CAD build for the part. Positions are in the model's coordinates, mm. A direction names the side the tool comes from. Give positions to 0.01 mm unless a question says otherwise; leave off trailing zeros. Order: outer loops, then holes, each group sorted by start corner. A loop starts at its lowest first (then second) coordinate and runs counter-clockwise, first axis right, second up.
```python
from build123d import *

# Parameters (mm, degrees)
BOSS_EXTRUDE1_DEPTH = 4.35
BOSS_EXTRUDE2_DEPTH = 22.8
CUT_EXTRUDE1_DEPTH  = 35.228241264
BOSS_EXTRUDE3_START = -12.57
SKETCH5_R           = 3.175
BOSS_EXTRUDE3_DEPTH = 12.57
SKETCH6_R           = 2.95
BOSS_EXTRUDE4_DEPTH = 2.6
CHAMFER1_SIZE       = 1.5
SKETCH7_R           = 1.5
CUT_EXTRUDE2_DEPTH  = 26.053852665
SKETCH8_R           = 1.25
CUT_EXTRUDE3_DEPTH  = 37.969425255
SKETCH9_W           = 15
SKETCH9_H           = 8.6
CUT_EXTRUDE4_DEPTH  = 25.4
CHAMFER2_SIZE       = 2.5
FILLET1_R           = 0.25


with BuildPart() as part:
    # Sketch2 → Boss-Extrude1 (new body)
    with BuildSketch(Plane(origin=(0, 0, 0), x_dir=(1, 0, 0), z_dir=(0, 1, 0))):
        with BuildLine():
            ThreePointArc((1.475, -16), (-1.7, -12.825), (-4.875, -16))
            Line((-4.875, -16), (1.475, -16))
        make_face()
        with BuildLine():
            Line((1.475, -16), (-4.875, -16))
            ThreePointArc((-4.875, -16), (-1.7, -19.175), (1.475, -16))
        make_face()
        with BuildLine():
            Line((-5.7, 15.863484846), (-5.7, 6.8))
            Line((-5.7, 6.8), (-5.7, -16))
            Line((-5.7, -16), (-4.875, -16))
            ThreePointArc((-4.875, -16), (-1.7, -12.825), (1.475, -16))
            Line((1.475, -16), (5.7, -16))
            Line((5.7, -16), (5.7, 6.8))
            Line((5.7, 6.8), (1.660846582, 14.02808686))
            ThreePointArc((1.660846582, 14.02808686), (0.248315373, 15.470627532), (-1.7, 16))
            Line((-1.7, 16), (-4.6, 16))
            ThreePointArc((-4.6, 16), (-5.154219358, 15.965740801), (-5.7, 15.863484846))
        make_face()
        with BuildLine():
            Line((-9.1, 6.8), (-5.7, 6.8))
            Line((-5.7, 6.8), (-5.7, 15.863484846))
            ThreePointArc((-5.7, 15.863484846), (-8.14964787, 14.265863337), (-9.1, 11.5))
            Line((-9.1, 11.5), (-9.1, 6.8))
        make_face()
    extrude(amount=BOSS_EXTRUDE1_DEPTH)

    # Sketch3 → Boss-Extrude2 (add)
    with BuildSketch(Plane.XY.offset(16)):
        with BuildLine():
            Line((5.7, 0.79), (-4.875, 4.092368421))
            Line((-4.875, 4.092368421), (-4.875, 2.831147875))
            ThreePointArc((-4.875, 2.831147875), (-1.758813758, 1.290370349), (-0.5, -1.95))
            ThreePointArc((-0.5, -1.95), (-0.966901247, -4.015007311), (-2.276772998, -5.678283585))
            Line((-2.276772998, -5.678283585), (5.7, 0.79))
        make_face()
        with BuildLine():
            ThreePointArc((-5.7, 2.833304297), (-7.287324911, 2.419272216), (-8.642534504, 1.494918444))
            ThreePointArc((-8.642534504, 1.494918444), (-8.890152665, -5.136032618), (-2.276772998, -5.678283585))
            ThreePointArc((-2.276772998, -5.678283585), (-0.966901247, -4.015007311), (-0.5, -1.95))
            ThreePointArc((-0.5, -1.95), (-1.758813758, 1.290370349), (-4.875, 2.831147875))
            Line((-4.875, 2.831147875), (-4.875, 0))
            Line((-4.875, 0), (-5.7, 0))
            Line((-5.7, 0), (-5.7, 2.833304297))
        make_face()
        with BuildLine():
            ThreePointArc((-4.875, 2.831147875), (-5.287453585, 2.849983603), (-5.7, 2.833304297))
            Line((-5.7, 2.833304297), (-5.7, 0))
            Line((-5.7, 0), (-4.875, 0))
            Line((-4.875, 0), (-4.875, 2.831147875))
        make_face()
        with BuildLine():
            Line((-4.875, 4.092368421), (-5.7, 4.35))
            Line((-5.7, 4.35), (-5.7, 2.833304297))
            ThreePointArc((-5.7, 2.833304297), (-5.287453585, 2.849983603), (-4.875, 2.831147875))
            Line((-4.875, 2.831147875), (-4.875, 4.092368421))
        make_face()
        with BuildLine():
            Line((-5.7, 2.833304297), (-5.7, 4.35))
            Line((-5.7, 4.35), (-8.642534504, 1.494918444))
            ThreePointArc((-8.642534504, 1.494918444), (-7.287324911, 2.419272216), (-5.7, 2.833304297))
        make_face()
    extrude(amount=-BOSS_EXTRUDE2_DEPTH)

    # Sketch4 → Cut-Extrude1 (cut, through all)
    with BuildSketch(Plane.XY.offset(16)):
        Polygon((5.7, 0), (5.7, 0.79), (4.725761535, 0), align=None)
    extrude(amount=-CUT_EXTRUDE1_DEPTH, mode=Mode.SUBTRACT)

    # Sketch5 → Boss-Extrude3 (add)
    with BuildSketch(Plane(origin=(0, 4.35, 0), x_dir=(1, 0, 0), z_dir=(0, 1, 0)).offset(BOSS_EXTRUDE3_START)):
        with Locations(Location((-1.7, -16, 0), (0, 0, 100.46651796))):
            Circle(SKETCH5_R)
    extrude(amount=BOSS_EXTRUDE3_DEPTH)

    # Sketch6 → Boss-Extrude4 (add)
    with BuildSketch(Plane.XY.offset(16)):
        with Locations((-5.3, -1.95)):
            Circle(SKETCH6_R)
    extrude(amount=BOSS_EXTRUDE4_DEPTH)

    # Chamfer1
    # the kernel refuses this chamfer: 1.5 mm, written as the material it takes off along each edge
    with BuildSketch(Plane(origin=(-5.273011582, -8.107902789, -6.8), x_dir=(0.017317974295388713, -0.021356755298707605, 0.9996219169112968), z_dir=(0.7767257469610731, 0.6298389587884852, 0))) as chamfer1_piece_1_section:
        Polygon((CHAMFER1_SIZE * 0.999621916911, -CHAMFER1_SIZE * 0.0274958766106), (-CHAMFER1_SIZE * 0.0274958766106, -CHAMFER1_SIZE * 0.999621916911), (0, 0), align=None)
    chamfer1_piece_1 = extrude(amount=16.730502051, mode=Mode.PRIVATE)
    chamfer1_piece_1 = split(chamfer1_piece_1, bisect_by=Plane(origin=(-2.677352376, 0, -6.368001428), z_dir=(0, -1, 0)), keep=Keep.TOP, mode=Mode.PRIVATE)
    add(chamfer1_piece_1, mode=Mode.SUBTRACT)

    # Sketch7 → Cut-Extrude2 (cut, through all)
    with BuildSketch(Plane(origin=(0, 4.35, 0), x_dir=(1, 0, 0), z_dir=(0, 1, 0))):
        with Locations(Location((-1.7, 12.15, 0), (0, 0, 270))):
            Circle(SKETCH7_R)
        with Locations(Location((-1.7, -16, 0), (0, 0, 270))):
            Circle(SKETCH7_R)
    extrude(amount=-CUT_EXTRUDE2_DEPTH, mode=Mode.SUBTRACT)

    # Sketch8 → Cut-Extrude3 (cut, through all)
    with BuildSketch(Plane.XY.offset(18.6)):
        with Locations((-5.3, -1.95)):
            Circle(SKETCH8_R)
    extrude(amount=-CUT_EXTRUDE3_DEPTH, mode=Mode.SUBTRACT)

    # Sketch9 → Cut-Extrude4 (cut)
    with BuildSketch(Plane(origin=(3.7, 0, 0), x_dir=(0, 0, -1), z_dir=(1, 0, 0))):
        with Locations((-4.814141793, -2.45)):
            Rectangle(SKETCH9_W, SKETCH9_H)
    extrude(amount=-CUT_EXTRUDE4_DEPTH, mode=Mode.SUBTRACT)

    # Chamfer2
    chamfer2_edges = [part.edges().sort_by_distance(p)[0] for p in [
        (3.7, 1.85, 4.814141793),
    ]]
    chamfer(chamfer2_edges, length=CHAMFER2_SIZE)

    # Fillet1
    # the kernel refuses this fillet: 0.25 mm, written as the material it takes off along each edge
    with BuildSketch(Plane(origin=(3.7, -0.831779531, 12.314141793), x_dir=(0, 1, 0), z_dir=(0, 0, -1))) as fillet1_piece_1:
        with BuildLine():
            CenterArc((0.408056999, 0.106294437), FILLET1_R, 140.961757793, 64.20015701)
            Line((0.213875562, 0.263754177), (0, 0))
            Line((0, 0), (0.181779531, 0))
        make_face()
    extrude(amount=15, mode=Mode.SUBTRACT)


with BuildPart() as body_2:
    # Mirror1: mirrored copy
    add(part.part.mirror(Plane.ZX.offset(4.35)))


solid = body_2.part
```
Item 1: Drop flat-ended pins along their axis: pin 1 Ø2.5 at (x, y) = (0, 13) entering from +Z; pin 2 Ø6 at (y, z) = (6.5, -9.5) entering from +X; pin 3 Ø3.5 at (x, z) = (-1.7, -12.15) entering from +Y; pin 4 Ø2.5 at (x, y) = (-2.5, 13.5) entering from -Z. Give the stop position or say it passes through.
Item 2: Slice it at A-A (y = 12.5). Give the cut face in (x, z) (3 decimals), and give its area (3 significant figures).
Item 3: Wall check: L1, parallel to Z at x = -6.25, y = 9.25; L2, parallel to X at y = 9.75, z = 15.5; L3, parallel to Y at x = -5.3, z = 14.75. Give the ranges that are in metal, low to high.
Item 4: Tool access for faces 4 (the face through (-3, 6.85, 5)), 5 (the face through (4, 7, 16)), 6 (the face through (-9, 10, 16)), 7 (the face through (-7, 11, 18.6)): list every direction of +Z, -Z, +X, -X, +Y, -Y with a clear straight run to the whole face (end or side of a thin tool).
Item 5: Slice it at D-D (z = -12.15). Give the cut face in (x, y), and give its area (3 significant figures).
Item 6: Two-plate mould, pull along X, no slides. Class faces 1 (the face through (-8, 5, -6.8)), 2 (the face through (0.27, 6.56, -15.46)), 3 (the face through (-1.63, 10.55, 14.5)): released by +X, released by -X, zero draft, split by the parting line, or undercut.
Item 7: Slice it at B-B (z = -4.5). Give the cut face in (x, y).
Item 8: Slice it at C-C (y = 10.65). Give the cut face in (x, z) (3 decimals), and give its area (3 significant figures).
A:
1. pin 1: stops at z = 19.14
1. pin 2: stops at x = 5.7
1. pin 3: stops at y = 8.7
1. pin 4: stops at z = -6.8
2. outline: (-9.729, -6.8) - (-2.342, -6.8) - (0.04, -5.3) - (0.04, -2.686) - (-9.729, -2.686) - close; (-9.729, 12.314) - (0.04, 12.314) - (0.04, 13.344) arc R3.175 ccw (long way) to (-3.522, 18.6) - (-7.598, 18.6) - (-7.598, 16) - (-9.729, 16) - close; hole circle Ø3 at (-1.7, 16)
2. area: 94.0 mm2
3. L1: z = -6.8 to -2.69, 12.31 to 18.6
3. L2: x = -10.01 to -6.17, -4.43 to -3.11, -0.29 to 3.43
3. L3: y = 4.35 to 9.4, 11.9 to 15.45
4. face 4: -X, +Y
4. face 5: +Z, +X, +Y, -Y
4. face 6: +Z, -X
4. face 7: +Z, -X, +Y, -Y
5. outline: (-9.05, 4.35) - (-3.2, 4.35) - (-3.2, 8.7) - (-9.05, 8.7) - close; (-0.2, 4.35) - (2.71, 4.35) - (2.71, 8.7) - (-0.2, 8.7) - close
5. area: 38.1 mm2
6. face 1: zero draft
6. face 2: released by +X
6. face 3: undercut
7. outline: (-8.64, 7.21) - (-5.7, 4.35) - (5.7, 4.35) - (5.7, 7.91) - (-2.28, 14.38) arc R4.8 ccw to start; hole circle Ø2.5 at (-5.3, 10.65)
8. outline: (-10.1, -6.8) - (-6.55, -6.8) - (-6.55, -2.686) - (-10.1, -2.686) - close; (-10.1, 12.314) - (-6.55, 12.314) - (-6.55, 18.6) - (-8.25, 18.6) - (-8.25, 16) - (-10.1, 16) - close; (-4.05, -6.8) - (-0.061, -6.8) - (2.321, -5.3) - (2.321, -2.686) - (-4.05, -2.686) - close; (-4.05, 12.314) - (2.321, 12.314) - (2.321, 16) - (1.475, 16) arc R3.175 ccw to (-3.522, 18.6) - (-4.05, 18.6) - close; hole circle Ø3 at (-1.7, 16)
8. area: 87.7 mm2
